Geometry check sheet. Reference: the model listing, model coordinates, mm. Face numbers are marked on the shaded views. A direction names the side the tool comes from. Round coordinates to 2 decimals unless told otherwise and drop trailing zeros. Write each loop counter-clockwise with the first axis right and the second up, starting at its lowest first coordinate (ties: lowest second). Pieces come first, ordered by that corner, then holes. Notation, with made-up numbers: (56.25, -35) -> (74.25, -35) arc R19 ccw to (74.25, -9) -> close; hole circle Ø3 at (75, -17). An arc over 180 degrees is marked (long way). Put each result on its own line as item: value. Start each with the question number.
from build123d import *

# Parameters (mm, degrees)
F0_W         = 35
F0_H         = 110
F1_DEPTH     = 3
F2_W         = 41
F2_H         = 116
F2_W_2       = 35
F2_H_2       = 110
F3_DEPTH     = 25
F4_R         = 1
F5_T1_DEPTH  = 30
F5_T4_ANGLE  = 90
F5_T6_ANGLE  = 90
F5_T8_ANGLE  = 90
F5_T10_ANGLE = 90
F7_W         = 100
F7_H         = 1
F8_DEPTH     = 1
F9_R         = 2


# Not quite as in the source:
# - a fillet or chamfer that OpenCascade refuses, or shapes differently, is made with other operations: its cross-section is extruded or revolved along the edge and cut away or added


with BuildPart() as f1:
    # F0 (on Top) → F1 (new body)
    with BuildSketch(Plane.XY):
        Rectangle(F0_W, F0_H)
    extrude(amount=F1_DEPTH)

    # F2 (on Top) → F3 (join)
    with BuildSketch(Plane.XY):
        Rectangle(F2_W, F2_H)
        Rectangle(F2_W_2, F2_H_2, mode=Mode.SUBTRACT)
    extrude(amount=F3_DEPTH)

    # F4
    f4_edges = [f1.edges().sort_by_distance(p)[0] for p in [
        (20.5, 0, 25),
        (0, 58, 25),
        (-20.5, 0, 25),
        (0, -58, 25),
        (-17.5, 0, 25),
        (0, 55, 25),
        (17.5, 0, 25),
        (0, -55, 25),
    ]]
    fillet(f4_edges, radius=F4_R)

    # F5: fillet of radius 2 on 4 edges, made by hand

    # F5_s2 → F5_t1 (cut)
    with BuildSketch(Plane.XY.offset(-5)):
        with BuildLine():
            ThreePointArc((20.5, -56), (19.9142135624, -57.4142135624), (18.5, -58))
            Line((18.5, -58), (20.5, -58))
            Line((20.5, -58), (20.5, -56))
        make_face()
        with BuildLine():
            ThreePointArc((-18.5, -58), (-19.9142135624, -57.4142135624), (-20.5, -56))
            Line((-20.5, -56), (-20.5, -58))
            Line((-20.5, -58), (-18.5, -58))
        make_face()
        with BuildLine():
            ThreePointArc((-18.5, 58), (-19.9142135624, 57.4142135624), (-20.5, 56))
            Line((-20.5, 56), (-20.5, 58))
            Line((-20.5, 58), (-18.5, 58))
        make_face()
        with BuildLine():
            ThreePointArc((20.5, 56), (19.9142135624, 57.4142135624), (18.5, 58))
            Line((18.5, 58), (20.5, 58))
            Line((20.5, 58), (20.5, 56))
        make_face()
    extrude(amount=F5_T1_DEPTH, mode=Mode.SUBTRACT)

    # F5_s3 → F5_t4 (revolve, cut)
    with BuildSketch(Plane.XZ.offset(-56)):
        with BuildLine():
            ThreePointArc((19.5, 25), (20.2071067812, 24.7071067812), (20.5, 24))
            Line((20.5, 24), (20.5, 25))
            Line((20.5, 25), (19.5, 25))
        make_face()
    revolve(axis=Axis((18.5, 56, 25), (0, 0, 1)), revolution_arc=F5_T4_ANGLE, mode=Mode.SUBTRACT)

    # F5_s5 → F5_t6 (revolve, cut)
    with BuildSketch(Plane.YZ.offset(-18.5)):
        with BuildLine():
            ThreePointArc((57, 25), (57.7071067812, 24.7071067812), (58, 24))
            Line((58, 24), (58, 25))
            Line((58, 25), (57, 25))
        make_face()
    revolve(axis=Axis((-18.5, 56, 25), (0, 0, 1)), revolution_arc=F5_T6_ANGLE, mode=Mode.SUBTRACT)

    # F5_s7 → F5_t8 (revolve, cut)
    with BuildSketch(Plane.XZ.offset(56)):
        with BuildLine():
            ThreePointArc((-19.5, 25), (-20.2071067812, 24.7071067812), (-20.5, 24))
            Line((-20.5, 24), (-20.5, 25))
            Line((-20.5, 25), (-19.5, 25))
        make_face()
    revolve(axis=Axis((-18.5, -56, 25), (0, 0, 1)), revolution_arc=F5_T8_ANGLE, mode=Mode.SUBTRACT)

    # F5_s9 → F5_t10 (revolve, cut)
    with BuildSketch(Plane.YZ.offset(18.5)):
        with BuildLine():
            ThreePointArc((-57, 25), (-57.7071067812, 24.7071067812), (-58, 24))
            Line((-58, 24), (-58, 25))
            Line((-58, 25), (-57, 25))
        make_face()
    revolve(axis=Axis((18.5, -56, 25), (0, 0, 1)), revolution_arc=F5_T10_ANGLE, mode=Mode.SUBTRACT)

    # F7 (on face) → F8 (cut)
    with BuildSketch(Plane(origin=(-20.5, 0, 0), x_dir=(0, -1, 0), z_dir=(-1, 0, 0))):
        with Locations((-0.0301606953, 18.6210061312)):
            Rectangle(F7_W, F7_H)
    extrude(amount=-F8_DEPTH, mode=Mode.SUBTRACT)

    # F9
    f9_edges = [f1.edges().sort_by_distance(p)[0] for p in [
        (19.914214, -57.414214, 0),
        (0, -58, 0),
        (-19.914214, -57.414214, 0),
        (-20.5, 0, 0),
        (-19.914214, 57.414214, 0),
        (0, 58, 0),
        (19.914214, 57.414214, 0),
        (20.5, 0, 0),
    ]]
    fillet(f9_edges, radius=F9_R)


solid = f1.part
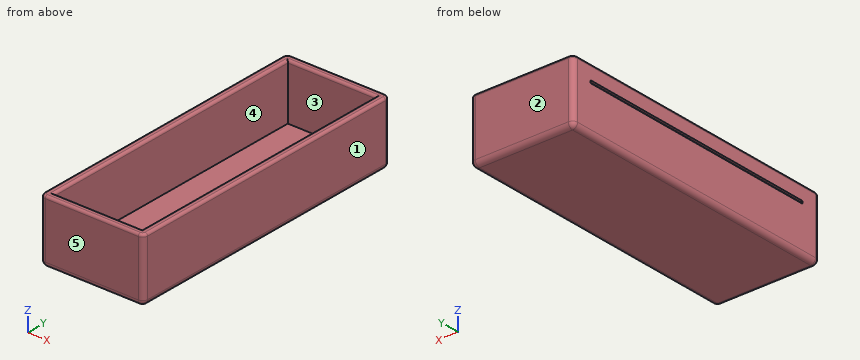
(1) Mould release check, pull along X, two halves, no side actions. Record for the marked faces 1, 2 and 3: +X half, -X half, draft (parallel to the pull), parting line (faces both ways), or undercut.
(2) Sectioned sample at B-B (y = 11). Record the cut outline in (x, z), and give its area (3 significant figures).
(3) Go/stop test with flat-tipped pins: pin 1 Ø1.1 at (x, z) = (-20, 19) entering from -Y; pin 2 Ø1.1 at (x, y) = (-20, -5) entering from -Z; pin 3 Ø2 at (y, z) = (-27.5, 18.5) entering from -X; pin 4 Ø4 at (x, y) = (3, 35) entering from +Z. Record where each tip stops, or that it passes through.
(4) Sectioned sample at A-A (z = 12.25). Record the cut outline in (x, y).
(5) Sectioned sample at C-C (x = -6.5). Record the cut outline in (y, z), and give its area (3 significant figures).
(6) Set-up check for the marked faces 4 and 5: record each of +Z, -Z, +X, -X, +Y, -Y from which the full face is reachable in a straight line by a thin tool's end or side.
(7) Material ranges on L1, parallel to Y at x = 15, z = 23.25; L2, parallel to X at y = -5.5, z = 7.25; L3, parallel to Z at x = 14.5, y = -31, recorded low to high. Write a range as from..to.
Found:
1. face 1: +X half
1. face 2: draft
1. face 3: undercut
2. outline: (-20.5, 2) arc R2 ccw to (-18.5, 0) -> (18.5, 0) arc R2 ccw to (20.5, 2) -> (20.5, 24) arc R1 ccw to (19.5, 25) -> (18.5, 25) arc R1 ccw to (17.5, 24) -> (17.5, 3) -> (-17.5, 3) -> (-17.5, 24) arc R1 ccw to (-18.5, 25) -> (-19.5, 25) arc R1 ccw to (-20.5, 24) -> (-20.5, 19.12) -> (-19.5, 19.12) -> (-19.5, 18.12) -> (-20.5, 18.12) -> close
2. area: 251 mm2
3. pin 1: y = -57.76
3. pin 2: z = 0.24
3. pin 3: x = -20.5
3. pin 4: z = 3
4. outline: (-20.5, -56) arc R2 ccw to (-18.5, -58) -> (18.5, -58) arc R2 ccw to (20.5, -56) -> (20.5, 56) arc R2 ccw to (18.5, 58) -> (-18.5, 58) arc R2 ccw to (-20.5, 56) -> close; hole (-17.5, -55) -> (17.5, -55) -> (17.5, 55) -> (-17.5, 55) -> close
5. outline: (-58, 2) arc R2 ccw to (-56, 0) -> (56, 0) arc R2 ccw to (58, 2) -> (58, 24) arc R1 ccw to (57, 25) -> (56, 25) arc R1 ccw to (55, 24) -> (55, 3) -> (-55, 3) -> (-55, 24) arc R1 ccw to (-56, 25) -> (-57, 25) arc R1 ccw to (-58, 24) -> close
5. area: 477 mm2
6. face 4: +Z
6. face 5: +Z, -Z, +X, -X, -Y
7. L1: -58..-55, 55..58
7. L2: -20.5..-17.5, 17.5..20.5
7. L3: 0..3
